Work out the finished part from the listing and answer in its coordinate system (mm). A direction names the side the tool comes from. Coordinates: 2 decimals unless noted, no trailing zeros. Order: outer loops, then holes, each group sorted by start corner. A loop starts at its lowest first (then second) coordinate and runs counter-clockwise, first axis right, second up. Notation, with made-up numbers: M 74,11 L 112,11 A21 cw 112,48 Z; hole C 13.25,-36.5 d11. An arc over 180 degrees is marked long. Answer in a Markdown table with one row per item. Add a question column.
Item 1: The mould has two halves that part along Y. Classify faces 6 (the face through (236.665, 0.117, 2.507)), 7 (the face through (135, -8.333, 0)), 8 (the face through (246, 3, -5)): released by +Y, released by -Y, zero draft, split by the parting line, or undercut.
Item 2: Flat-ended cylindrical pins translate along their axes: pin 1 Ø0.8 at (x, z) = (140.5, -2.5) entering from +Y; pin 2 Ø0.5 at (x, z) = (182, -2.5) entering from -Y; pin 3 Ø3 at (x, z) = (253.5, -1.5) entering from +Y. Find the tip coordinate at first contact, or state that the pin passes through.
Item 3: The part is cut by section B-B (x = 38). Write down the section's boundary in (y, z).
Item 4: Which of the six approach directions +Z, -Z, +X, -X, +Y, -Y give full straight-line access (tool end or side, diameter ignored) to faces 1 (the face through (236.665, 0.117, -2.493)), 2 (the face through (138, 8.333, 0)), 3 (the face through (8, 2.34, 0.07)), 4 (the face through (132, 0, 2)), 5 (the face through (238.387, -9.877, 0.042))?
Item 5: The part is cut by section A-A (x = 181). Write down the section's boundary in (y, z), then the cut area to 3 significant figures.
Item 6: Consider line 1 (X direction, y = 12.5, z = -1); line 2 (Y direction, x = 144, z = 2.5); line 3 (Y direction, x = 96.5, z = 1). Determine where each line is inside the solid, lowest interval first. Write a range as from..to.
from build123d import *

# Parameters (mm, degrees)
BOSS_EXTRUDE1_DEPTH   = 5
SKETCH1_R             = 16.666666667
BOSS_EXTRUDE1_2_DEPTH = 5
BOSS_EXTRUDE2_DEPTH   = 3
BOSS_EXTRUDE3_DEPTH   = 2


with BuildPart() as part:
    # Sketch1 → Boss-Extrude1 (new, symmetric)
    with BuildSketch(Plane.XY):
        with BuildLine():
            Line((-24.290235769, 5.914765107), (0.016914075, 12.427846278))
            ThreePointArc((0.016914075, 12.427846278), (8.049381886, 2.156825376), (6.228571158, -10.754373553))
            Line((6.228571158, -10.754373553), (-18.078578687, -17.267454724))
            ThreePointArc((-18.078578687, -17.267454724), (24.148145657, 6.470476128), (-24.290235769, 5.914765107))
        make_face()
    extrude(amount=BOSS_EXTRUDE1_DEPTH, both=True)



with BuildPart() as body_2:
    # Sketch1 → Boss-Extrude1 2 (new, symmetric)
    with BuildSketch(Plane.XY):
        with Locations((258.333333333, 0)):
            Circle(SKETCH1_R)
        Polygon((270.333333333, 3.215390309), (270.333333333, 6.92820323), (267.117943024, 8.784609691), (265.261536564, 12), (261.548723643, 12), (258.333333333, 13.856406461), (255.117943024, 12), (251.405130103, 12), (249.548723643, 8.784609691), (246.333333333, 6.92820323), (246.333333333, 3.215390309), (244.476926873, 0), (246.333333333, -3.215390309), (246.333333333, -6.92820323), (249.548723643, -8.784609691), (251.405130103, -12), (255.117943024, -12), (258.333333333, -13.856406461), (261.548723643, -12), (265.261536564, -12), (267.117943024, -8.784609691), (270.333333333, -6.92820323), (270.333333333, -3.215390309), (272.189739794, 0), align=None, mode=Mode.SUBTRACT)
    extrude(amount=BOSS_EXTRUDE1_2_DEPTH, both=True)


with BuildPart() as part_1:
    add(part.part)

    add(body_2.part)  # Boss-Extrude2 merges body 2
    # Sketch1_3 → Boss-Extrude2 (add, symmetric)
    with BuildSketch(Plane.XY):
        with BuildLine():
            ThreePointArc((47.140452079, 8.333333333), (30.473785412, 11.192881254), (15.713484026, 19.444444444))
            ThreePointArc((15.713484026, 19.444444444), (25, 0), (15.713484026, -19.444444444))
            ThreePointArc((15.713484026, -19.444444444), (30.473785412, -11.192881254), (47.140452079, -8.333333333))
            Line((47.140452079, -8.333333333), (226.058472115, -8.333333333))
            ThreePointArc((226.058472115, -8.333333333), (238.558472115, -9.921041506), (250.264618029, -14.583333333))
            ThreePointArc((250.264618029, -14.583333333), (241.666666667, 0), (250.264618029, 14.583333333))
            ThreePointArc((250.264618029, 14.583333333), (238.558472115, 9.921041506), (226.058472115, 8.333333333))
            Line((226.058472115, 8.333333333), (47.140452079, 8.333333333))
        make_face()
        with BuildLine():
            ThreePointArc((35.333333333, -5.333333333), (30, 0), (35.333333333, 5.333333333))
            Line((35.333333333, 5.333333333), (231.333333333, 5.333333333))
            ThreePointArc((231.333333333, 5.333333333), (236.666666667, 0), (231.333333333, -5.333333333))
            Line((231.333333333, -5.333333333), (35.333333333, -5.333333333))
        make_face(mode=Mode.SUBTRACT)
    extrude(amount=BOSS_EXTRUDE2_DEPTH, both=True)

    # Sketch1_4 → Boss-Extrude3 (add, symmetric)
    with BuildSketch(Plane.XY):
        with BuildLine():
            Line((35.333333333, -5.333333333), (231.333333333, -5.333333333))
            ThreePointArc((231.333333333, -5.333333333), (236.666666667, 0), (231.333333333, 5.333333333))
            Line((231.333333333, 5.333333333), (35.333333333, 5.333333333))
            ThreePointArc((35.333333333, 5.333333333), (30, 0), (35.333333333, -5.333333333))
        make_face()
    extrude(amount=BOSS_EXTRUDE3_DEPTH, both=True)


solid = part_1.part
Reply:
| question | item | result |
|---|---|---|
| 1 | face 6 | undercut |
| 1 | face 7 | released by -Y |
| 1 | face 8 | zero draft |
| 2 | pin 1 | stops at y = 8.33 |
| 2 | pin 2 | stops at y = -8.33 |
| 2 | pin 3 | stops at y = 16.33 |
| 3 | outline | M -9.18,-3 L -5.33,-3 L -5.33,-2 L 5.33,-2 L 5.33,-3 L 9.18,-3 L 9.18,3 L 5.33,3 L 5.33,2 L -5.33,2 L -5.33,3 L -9.18,3 Z |
| 4 | face 1 | -Z |
| 4 | face 2 | +Z, -Z, +Y |
| 4 | face 3 | +Z, -Z |
| 4 | face 4 | +Z |
| 4 | face 5 | +Z, -Z, -Y |
| 5 | outline | M -8.33,-3 L -5.33,-3 L -5.33,-2 L 5.33,-2 L 5.33,-3 L 8.33,-3 L 8.33,3 L 5.33,3 L 5.33,2 L -5.33,2 L -5.33,3 L -8.33,3 Z |
| 5 | area | 78.7 mm2 |
| 6 | line 1 | x = -21.65..27.16, 246.04..255.98, 260.68..269.36 |
| 6 | line 2 | y = -8.33..-5.33, 5.33..8.33 |
| 6 | line 3 | y = -8.33..8.33 |
